Part model, mm, in its own coordinate system. Face numbers are marked on the shaded views. A direction names the side the tool comes from. Give positions to 0.01 mm unless a question says otherwise; leave off trailing zeros. Order: outer loops, then holes, each group sorted by start corner. A loop starts at its lowest first (then second) coordinate and runs counter-clockwise, first axis right, second up.
1. Probe line 1 (Z direction, x = 0, y = 10.25); line 2 (Y direction, x = 3, z = 0.75); line 3 (X direction, y = 25.25, z = -1). List the from-to ranges inside material, lowest first.
2. Slice it at D-D on z = 2.5. List the corners of the cut face in (x, y).
3. Which spindle directions (+Z, -Z, +X, -X, +Y, -Y) get a long thin tool onto all of the face, cutting with end or side? Do the marked faces 1, 2 and 3. Say none if no direction does.
4. Slice it at A-A on x = 0. List the corners of the cut face in (y, z).
5. Slice it at B-B on y = 7.25. List the corners of the cut face in (x, z), and give its area (3 significant figures).
6. Slice it at C-C on z = 0.75. List the corners of the cut face in (x, y), and give its area (3 significant figures).
7. Drop flat-ended pins along their axis: pin 1 Ø1.5 at (y, z) = (25.5, -0.5) entering from -X; pin 2 Ø3 at (x, y) = (2, 12.5) entering from +Z; pin 3 Ø0.9 at (x, z) = (-0.5, 0.5) entering from -Y. Give the stop position or say it passes through.
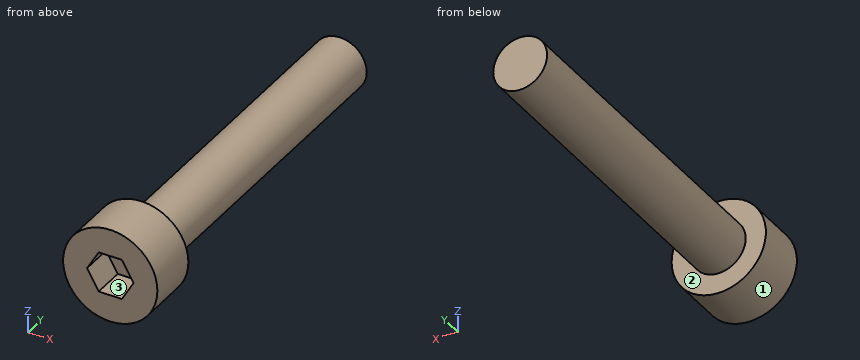
from build123d import *

# Parameters (mm, degrees)
SKETCH_1_R          = 3.5
EXTRUDE_1_DEPTH     = 3.9
SKETCH_2_R          = 2
EXTRUDE_2_DEPTH     = 25
CUT_EXTRUDE_1_DEPTH = 2.4


with BuildPart() as part:
    # 草图1 → 凸台-拉伸1 (new body)
    with BuildSketch(Plane(origin=(0, 0, 0), x_dir=(1, 0, 0), z_dir=(0, 1, 0))):
        Circle(SKETCH_1_R)
    extrude(amount=EXTRUDE_1_DEPTH)

    # 草图2 → 凸台-拉伸2 (add)
    with BuildSketch(Plane(origin=(0, 3.9, 0), x_dir=(1, 0, 0), z_dir=(0, 1, 0))):
        Circle(SKETCH_2_R)
    extrude(amount=EXTRUDE_2_DEPTH)

    # 草图3 → 切除-拉伸1 (cut)
    with BuildSketch(Plane.XZ):
        Polygon((1.725, 0), (0.8625, 1.493893822), (-0.8625, 1.493893822), (-1.725, 0), (-0.8625, -1.493893822), (0.8625, -1.493893822), align=None)
    extrude(amount=-CUT_EXTRUDE_1_DEPTH, mode=Mode.SUBTRACT)


solid = part.part
Data:
1. line 1: z = -2 to 2
1. line 2: y = 0 to 3.9
1. line 3: x = -1.73 to 1.73
2. outline: (-2.45, 0) - (2.45, 0) - (2.45, 3.9) - (-2.45, 3.9) - close
3. face 1: +Y, -Y
3. face 2: +Y
3. face 3: -Y
4. outline: (0, -3.5) - (3.9, -3.5) - (3.9, -2) - (28.9, -2) - (28.9, 2) - (3.9, 2) - (3.9, 3.5) - (0, 3.5) - (0, 1.49) - (2.4, 1.49) - (2.4, -1.49) - (0, -1.49) - close
5. outline: circle Ø4 at (0, 0)
5. area: 12.6 mm2
6. outline: (-3.42, 0) - (-1.29, 0) - (-1.29, 2.4) - (1.29, 2.4) - (1.29, 0) - (3.42, 0) - (3.42, 3.9) - (1.85, 3.9) - (1.85, 28.9) - (-1.85, 28.9) - (-1.85, 3.9) - (-3.42, 3.9) - close
6. area: 113 mm2
7. pin 1: stops at x = -2
7. pin 2: stops at z = 1.94
7. pin 3: stops at y = 2.4
